Work out the finished part from the listing and answer in its coordinate system (mm). Coordinates: 2 decimals unless noted, no trailing zeros. Order: outer loops, then holes, each group sorted by start corner. A loop starts at its lowest first (then second) coordinate and runs counter-clockwise, first axis right, second up. Notation, with made-up numbers: (-6, 31) -> (36, 31) arc R12 ccw to (36, 50) -> close; hole circle Ø1 at (74, -2.5). An arc over 180 degrees is marked (long way). Answer as CSV lines item,"result". Start each with the question number.
Item 1: Section C-C (x = 0.35) is taken. Write down the section's boundary in (y, z).
Item 2: Section A-A (z = 13) is taken. Write down the section's boundary in (x, y).
Item 3: Straight lines are drawn through the part: L1, parallel to Y at x = 0.5, z = -10; L2, parallel to Z at x = 0.95, y = -13.5; L3, parallel to Y at x = 0.65, z = -16.5. For each, find the intervals that lie inside material, in ascending order.
Item 4: Each of these flat-tipped pins is pushed along its axis until it touches: pin 1 Ø3.5 at (y, z) = (-8, -10) entering from +X; pin 2 Ø1.5 at (y, z) = (-90.5, -6.5) entering from -X. Where does it stop, or does it pass through?
Item 5: Section B-B (y = -8) is taken. Write down the section's boundary in (x, z).
```python
from build123d import *

# Parameters (mm, degrees)
SKETCH1_W                = 36
SKETCH1_H                = 110
BOSS_EXTRUDE1_DEPTH      = 1
F_4_0_4_DIAMETER_HOLE2_D = 4
F_4_0_4_DIAMETER_HOLE3_D = 4
BOSS_EXTRUDE2_DEPTH      = 1
FILLET1_R                = 4
FILLET2_R                = 4


with BuildPart() as part:
    # Sketch1 → Boss-Extrude1 (new body)
    with BuildSketch(Plane(origin=(0, 0, 0), x_dir=(0, 0, -1), z_dir=(1, 0, 0))):
        with Locations((0, -55)):
            Rectangle(SKETCH1_W, SKETCH1_H)
    extrude(amount=BOSS_EXTRUDE1_DEPTH)

    # Ø4.0 (4) Diameter Hole2 (through all)
    with Locations(Plane.ZY):
        with Locations((-10, -8), (10, -8)):
            Hole(F_4_0_4_DIAMETER_HOLE2_D / 2)

    # Ø4.0 (4) Diameter Hole3 (through all)
    with Locations(Plane.ZY):
        with Locations((-13, -17), (13, -17)):
            Hole(F_4_0_4_DIAMETER_HOLE3_D / 2)

    # Sketch9 → Boss-Extrude2 (add)
    with BuildSketch(Plane.ZY):
        Polygon((18, -23.35), (20, -25.35), (20, -110), (18, -110), align=None)
        Polygon((-18, -23.35), (-20, -25.35), (-20, -110), (-18, -110), align=None)
    extrude(amount=-BOSS_EXTRUDE2_DEPTH)

    # Fillet1
    fillet1_edges = [part.edges().sort_by_distance(p)[0] for p in [
        (0.5, 0, 18),
        (0.5, 0, -18),
    ]]
    fillet(fillet1_edges, radius=FILLET1_R)

    # Fillet2
    fillet2_edges = [part.edges().sort_by_distance(p)[0] for p in [
        (0.5, -25.35, 20),
        (0.5, -110, 20),
        (0.5, -110, -20),
        (0.5, -25.35, -20),
    ]]
    fillet(fillet2_edges, radius=FILLET2_R)


solid = part.part
```
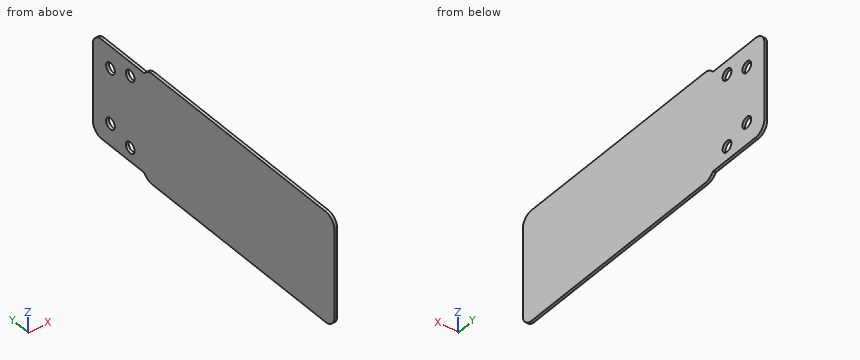
Checked values:
1,outline,"(-110, -16) arc R4 ccw to (-106, -20) -> (-27.01, -20) arc R4 ccw to (-24.18, -18.83) -> (-23.35, -18) -> (-4, -18) arc R4 ccw to (0, -14) -> (0, 14) arc R4 ccw to (-4, 18) -> (-23.35, 18) -> (-24.18, 18.83) arc R4 ccw to (-27.01, 20) -> (-106, 20) arc R4 ccw to (-110, 16) -> close; hole circle Ø4 at (-17, -13); hole circle Ø4 at (-17, 13); hole circle Ø4 at (-8, -10); hole circle Ø4 at (-8, 10)"
2,outline,"(0, -110) -> (1, -110) -> (1, -19) -> (0, -19) -> close; (0, -15) -> (1, -15) -> (1, 0) -> (0, 0) -> close"
3,L1,"y = -110 to -10, -6 to 0"
3,L2,"z = -18 to 18"
3,L3,"y = -109.97 to -0.88"
4,pin 1,"passes through"
4,pin 2,"stops at x = 0"
5,outline,"(0, -18) -> (1, -18) -> (1, -12) -> (0, -12) -> close; (0, -8) -> (1, -8) -> (1, 8) -> (0, 8) -> close; (0, 12) -> (1, 12) -> (1, 18) -> (0, 18) -> close"
